from build123d import *

# Parameters (mm, degrees)
F2_R = 6.096
F4_R = 1.27


# Not quite as in the source:
# - a fillet or chamfer that OpenCascade refuses, or shapes differently, is made with other operations: its cross-section is extruded or revolved along the edge and cut away or added


with BuildPart() as f1:
    # F0 (on Front) → F1 (revolve)
    with BuildSketch(Plane.XZ):
        Polygon((-25.6974867058, 3.96875), (-25.6974867058, 0), (37.8025132942, 0), (37.8025132942, 8.73125), (-19.3474867058, 8.73125), (-19.3474867058, 3.96875), align=None)
    revolve(axis=Axis((6.0525132942, 0, 0), (1, 0, 0)))

    # F2
    f2_edges = [f1.edges().sort_by_distance(p)[0] for p in [
        (37.802513, 0, -8.73125),
    ]]
    fillet(f2_edges, radius=F2_R)

    # F3: fillet of radius 7.62 on 1 edges, made by hand

    # F3_s1 → F3_t2 (revolve, cut)
    with BuildSketch(Plane.XZ):
        with BuildLine():
            ThreePointArc((-12.2835576468, 8.73125), (-16.543267144, 7.4294202256), (-19.3474867058, 3.96875))
            Line((-19.3474867058, 3.96875), (-19.3474867058, 8.73125))
            Line((-19.3474867058, 8.73125), (-12.2835576468, 8.73125))
        make_face()
    revolve(axis=Axis((-19.3474867058, 0, 0), (1, 0, 0)), mode=Mode.SUBTRACT)

    # F4
    f4_edges = [f1.edges().sort_by_distance(p)[0] for p in [
        (-22.522487, 0, 3.96875),
        (-25.697487, 0, -3.96875),
        (-19.347487, 0, -3.96875),
    ]]
    fillet(f4_edges, radius=F4_R)


solid = f1.part
Design review of the part built by this model. Coordinates are the model's own, in mm. A direction names the side the tool comes from. Coordinates: 2 decimals unless noted, no trailing zeros. Order: outer loops, then holes, each group sorted by start corner. A loop starts at its lowest first (then second) coordinate and runs counter-clockwise, first axis right, second up.
Item 1: For line 1 (Y direction, x = 22, z = 0.25); line 2 (Z direction, x = 27, y = -2.5); line 3 (X direction, y = 4.25, z = 4.5), list the stretches that pass through material, from the lowest coordinate up.
Item 2: For faces 1 (the cylindrical face through (-22.322, -1.192, 3.785)), 2 (the flat face through (-25.697, 0, 0)), list the 3-axis set-ups (+Z, -Z, +X, -X, +Y, -Y) from which the entire face can be reached by the end or side of a thin tool; tool diameter is ignored.
Item 3: Take a section at A-A, the plane x = -6. Write out the cut boundary in (y, z).
Item 4: For pin 1 Ø3 at (x, y) = (26.5, 3) entering from -Z; pin 2 Ø1 at (x, y) = (-11.5, -6.5) entering from +Z; pin 3 Ø1 at (y, z) = (-3, 2) entering from -X, all flat-tipped, find the tip position at first contact; note any pin that passes through.
Item 5: The part is to be moulded in two halves that separate along Y. For faces 3 (the cylindrical face through (9.4, 5.31, -6.93)), 4 (the flat face through (37.803, 0, 0)), say which applies: pulls with the +Y half, pulls with the -Y half, needs draft (parallel to the pull), parting line crosses it, or undercut.
The answers:
1. line 1: y = -8.73 to 8.73
1. line 2: z = -8.37 to 8.37
1. line 3: x = -17.96 to 36.66
2. face 1: -X
2. face 2: +Z, -Z, -X, +Y, -Y
3. outline: circle Ø17.46 at (0, 0)
4. pin 1: stops at z = -8.6
4. pin 2: stops at z = 6.34
4. pin 3: stops at x = -25.63
5. face 3: parting line crosses it
5. face 4: needs draft
